Work out the finished part from the listing and answer in its coordinate system (mm). Coordinates: 2 decimals unless noted, no trailing zeros. Order: outer loops, then holes, each group sorted by start corner. A loop starts at its lowest first (then second) coordinate and runs counter-clockwise, first axis right, second up. Notation, with made-up numbers: M 6,62 L 30,62 A7 cw 30,69 Z; hole C 65.5,-23.75 d7. An arc over 180 degrees is marked long. Answer in a Markdown table with one row per item. Add a question column.
Item 1: The part is cut by section A-A (x = 0). Write down the section's boundary in (y, z) (3 decimals).
Item 2: Consider line 1 (Y direction, x = -6.5, z = 2.5); line 2 (X direction, y = -35, z = 6.5); line 3 (X direction, y = 38, z = 4.25). Determine where each line is inside the solid, lowest interval first. Write a range as from..to.
Item 3: The part is cut by section C-C (z = 4). Write down the section's boundary in (x, y), then the cut area to 3 significant figures.
Item 4: The part is cut by section B-B (y = 0). Write down the section's boundary in (x, z) (3 decimals).
Item 5: The part is cut by section D-D (y = 17.5). State how many separate pieces and enclosed holes the cut face has, then the cut area to 3 significant figures.
Item 6: The mould has two halves that part along Y. Classify faces 1 (the face through (-1, 12, 0)), 2 (the face through (-5.411, -27, 5)), 3 (the face through (-9.31, 8.64, 5.01)), 4 (the face through (57.095, -2.513, 0.966)): released by +Y, released by -Y, zero draft, split by the parting line, or undercut.
Item 7: Flat-ended cylindrical pins translate along their axes: pin 1 Ø5 at (y, z) = (-22, 6) entering from +X; pin 2 Ø6 at (y, z) = (5.5, 8.5) entering from -X; pin 3 Ø3 at (y, z) = (25.5, 5) entering from +X. Find the tip coordinate at first contact, or state that the pin passes through.
from build123d import *

# Parameters (mm, degrees)
CUT_EXTRUDE2_DEPTH = 82.458397971
CUT_EXTRUDE3_DEPTH = 82.458397971


with BuildPart() as part:
    # Sketch1 → Revolve1 (revolve)
    with BuildSketch(Plane(origin=(0, 0, 0), x_dir=(1, 0, 0), z_dir=(0, 1, 0))):
        with BuildLine():
            Line((-57.15, 0), (-57.15, -1.905))
            ThreePointArc((-57.15, -1.905), (-53.975, -5.08), (-57.15, -8.255))
            Line((-57.15, -8.255), (-57.15, -10.16))
            Line((-57.15, -10.16), (0, -10.16))
            Line((0, -10.16), (0, 0))
            Line((0, 0), (-57.15, 0))
        make_face()
    revolve(axis=Axis((0, 0, 0), (0, 0, 1)))

    # Sketch3 → Cut-Extrude2 (cut, through all)
    with BuildSketch(Plane(origin=(0, 0, 0), x_dir=(-1, 0, 0), z_dir=(0, 0, -1))):
        with BuildLine():
            Line((6.35, 43.004116755), (6.35, 10.998522628))
            ThreePointArc((6.35, 10.998522628), (9.347244518, 8.597617108), (11.489808035, 5.410574028))
            Line((11.489808035, 5.410574028), (43.132380488, 5.410574028))
            ThreePointArc((43.132380488, 5.410574028), (31.071612581, 30.401175134), (6.35, 43.004116755))
        make_face()
        with BuildLine():
            Line((5.410574028, -11.489808035), (5.410574028, -43.132380488))
            ThreePointArc((5.410574028, -43.132380488), (30.401175134, -31.071612581), (43.004116755, -6.35))
            Line((43.004116755, -6.35), (10.998522628, -6.35))
            ThreePointArc((10.998522628, -6.35), (8.597617108, -9.347244518), (5.410574028, -11.489808035))
        make_face()
        with BuildLine():
            Line((-11.489808035, -5.410574028), (-43.132380488, -5.410574028))
            ThreePointArc((-43.132380488, -5.410574028), (-31.071612581, -30.401175134), (-6.35, -43.004116755))
            Line((-6.35, -43.004116755), (-6.35, -10.998522628))
            ThreePointArc((-6.35, -10.998522628), (-9.347244518, -8.597617108), (-11.489808035, -5.410574028))
        make_face()
        with BuildLine():
            Line((-5.410574028, 11.489808035), (-5.410574028, 43.132380488))
            ThreePointArc((-5.410574028, 43.132380488), (-30.401175134, 31.071612581), (-43.004116755, 6.35))
            Line((-43.004116755, 6.35), (-10.998522628, 6.35))
            ThreePointArc((-10.998522628, 6.35), (-8.597617108, 9.347244518), (-5.410574028, 11.489808035))
        make_face()
    extrude(amount=-CUT_EXTRUDE2_DEPTH, mode=Mode.SUBTRACT)

    # Sketch6 → Cut-Extrude3 (cut, through all)
    with BuildSketch(Plane(origin=(0, 0, 0), x_dir=(-1, 0, 0), z_dir=(0, 0, -1))):
        with BuildLine():
            Line((-2.794, 3.123786965), (-2.794, -3.123786965))
            ThreePointArc((-2.794, -3.123786965), (0, -4.191), (2.794, -3.123786965))
            Line((2.794, -3.123786965), (2.794, 3.123786965))
            ThreePointArc((2.794, 3.123786965), (0, 4.191), (-2.794, 3.123786965))
        make_face()
    extrude(amount=-CUT_EXTRUDE3_DEPTH, mode=Mode.SUBTRACT)


solid = part.part
Reply:
| question | item | result |
|---|---|---|
| 1 | outline | M -57.15,0 L -4.191,0 L -4.191,10.16 L -57.15,10.16 L -57.15,8.255 A3.175 cw -57.15,1.905 Z; M 4.191,0 L 57.15,0 L 57.15,1.905 A3.175 cw 57.15,8.255 L 57.15,10.16 L 4.191,10.16 Z |
| 2 | line 1 | y = -54.92..-42.98, -10.91..10.91, 42.98..54.92 |
| 2 | line 2 | x = -41.53..-25.78, -5.41..6.35, 25.78..41.53 |
| 2 | line 3 | x = -38.49..-21.11, -6.35..5.41, 21.11..38.49 |
| 3 | outline | C 0,0 d108.33; hole M -43.13,5.41 L -11.49,5.41 A12.7 cw -6.35,11 L -6.35,43 A43.47 ccw Z; hole M -43,-6.35 A43.47 ccw -5.41,-43.13 L -5.41,-11.49 A12.7 cw -11,-6.35 Z; hole M -2.79,-3.12 A4.19 ccw 2.79,-3.12 L 2.79,3.12 A4.19 ccw -2.79,3.12 Z; hole M 5.41,11.49 A12.7 cw 11,6.35 L 43,6.35 A43.47 ccw 5.41,43.13 Z; hole M 6.35,-43 A43.47 ccw 43.13,-5.41 L 11.49,-5.41 A12.7 cw 6.35,-11 Z |
| 3 | area | 5,210 mm2 |
| 4 | outline | M -57.15,0 L -2.794,0 L -2.794,10.16 L -57.15,10.16 L -57.15,8.255 A3.175 cw -57.15,1.905 Z; M 2.794,0 L 57.15,0 L 57.15,1.905 A3.175 cw 57.15,8.255 L 57.15,10.16 L 2.794,10.16 Z |
| 5 | separate pieces | 3 |
| 5 | enclosed holes | 0 |
| 5 | area | 383 mm2 |
| 6 | face 1 | zero draft |
| 6 | face 2 | undercut |
| 6 | face 3 | undercut |
| 6 | face 4 | split by the parting line |
| 7 | pin 1 | stops at x = 53.18 |
| 7 | pin 2 | stops at x = -57.1 |
| 7 | pin 3 | stops at x = 48.37 |
